The model under review builds one solid part; all positions refer to its coordinate system, in mm. Round coordinates to 2 decimals unless told otherwise and drop trailing zeros. Loops run counter-clockwise (first coordinate to the right, second up) from the corner with the lowest first, then second, coordinate; pieces in that order, holes last. Notation, with made-up numbers: (-3, 36) -> (15, 36) arc R21 cw to (15, 60) -> close; hole circle Ø6 at (-40, 34). An arc over 180 degrees is marked (long way). Use a Markdown table: item, result. Add a question column.
1) Consider section A-A on z = 0. Give the boundary of the cut face in (x, y), plus the area to 3 significant figures.
2) Insertion check: pin 1 (1.5 mm diameter, centred on x = -5, y = -2, fed in from -Z); pin 2 (2 mm diameter, centred on y = 1.5, z = 36, fed in from -X); pin 3 (2 mm diameter, centred on x = -2, z = 26.5, fed in from +Y). Each pin has a flat end and moves straight along its axis. Give the tip position at first contact, or say it passes through.
3) Wall thickness on probe 1 along X at (y, z) = (0.25, 0); probe 2 along Z at (x, y) = (0.25, 0.75); probe 3 along Z at (x, y) = (-2, -1.25): over which ranges is each line inside the solid? List them lowest first.
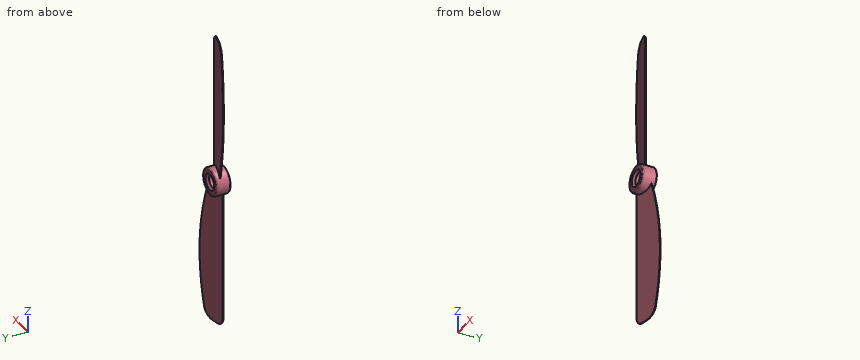
from build123d import *

# Parameters (mm, degrees)
SKETCH1_R           = 5.75
BOSS_EXTRUDE1_DEPTH = 3
BOSS_EXTRUDE2_DEPTH = 0.15
CIRPATTERN1_COUNT   = 2
SKETCH4_R           = 2.5
CUT_EXTRUDE1_DEPTH  = 7.0000001
FILLET1_R           = 0.5
CHAMFER1_SIZE       = 1


with BuildPart() as part:
    # Sketch1 → Boss-Extrude1 (new body, symmetric)
    with BuildSketch(Plane(origin=(0, 0, 0), x_dir=(1, 0, 0), z_dir=(0, 1, 0))):
        Circle(SKETCH1_R)
    extrude(amount=BOSS_EXTRUDE1_DEPTH, both=True)

    # Sketch3 → Boss-Extrude2 (add, symmetric)
    with BuildSketch(Plane(origin=(0, 0, 0), x_dir=(0.974370065, -0.224951054, 0), z_dir=(-0.224951054, -0.974370065, 0))):
        with BuildLine():
            add(Edge.make_bspline(
                [(3.543368809, 3.784271818), (1.869103712, 5.75), (-0.674853163, 5.75)],
                knots=[5.430726938, 5.430726938, 5.430726938, 6.283185307, 6.283185307, 6.283185307], degree=2, weights=[1, 0.910531227, 1]))
            Line((3.543368809, 3.784271818), (3.543368809, 60.5))
            ThreePointArc((3.543368809, 60.5), (2.664689152, 62.621320344), (0.543368809, 63.5))
            Line((0.543368809, 63.5), (-2.327174273, 63.5))
            ThreePointArc((-2.327174273, 63.5), (-5.459156928, 62.397522886), (-7.209963904, 59.576273859))
            add(Edge.make_bspline(
                [(-4.893075135, 3.784271818), (-10.655609146, 21.734523113), (-11.43974903, 40.386779673), (-7.209963904, 59.576273859)],
                knots=[0, 0, 0, 0, 0.936316624, 0.936316624, 0.936316624, 0.936316624], degree=3))
            add(Edge.make_bspline(
                [(-0.674853163, 5.75), (-3.218810038, 5.75), (-4.893075135, 3.784271818)],
                knots=[0, 0, 0, 0.852458369, 0.852458369, 0.852458369], degree=2, weights=[1, 0.910531227, 1]))
        make_face()
    boss_extrude2 = extrude(amount=BOSS_EXTRUDE2_DEPTH, both=True)

    # CirPattern1: Boss-Extrude2 ×2 about axis
    cirpattern1_axis = Axis((0, 3, 0), (0, -1, 0))
    for i in range(1, CIRPATTERN1_COUNT):
        add(boss_extrude2.rotate(cirpattern1_axis, i * 360 / CIRPATTERN1_COUNT))

    # Sketch4 → Cut-Extrude1 (cut, through all)
    with BuildSketch(Plane(origin=(0, 3, 0), x_dir=(1, 0, 0), z_dir=(0, 1, 0))):
        Circle(SKETCH4_R)
    extrude(amount=-CUT_EXTRUDE1_DEPTH, mode=Mode.SUBTRACT)

    # Fillet1
    fillet1_edges = [part.edges().sort_by_distance(p)[0] for p in [
        (-5.75, -3, 0),
        (-5.75, 3, 0),
    ]]
    fillet(fillet1_edges, radius=FILLET1_R)

    # Chamfer1
    chamfer1_edges = [part.edges().sort_by_distance(p)[0] for p in [
        (-2.5, -3, 0),
        (-2.5, 3, 0),
    ]]
    chamfer(chamfer1_edges, length=CHAMFER1_SIZE)


solid = part.part
Result set:
| question | item | result |
|---|---|---|
| 1 | outline | (-5.75, -2.5) arc R0.5 ccw to (-5.25, -3) -> (-3.5, -3) -> (-2.5, -2) -> (-2.5, 2) -> (-3.5, 3) -> (-5.25, 3) arc R0.5 ccw to (-5.75, 2.5) -> close; (2.5, -2) -> (3.5, -3) -> (5.25, -3) arc R0.5 ccw to (5.75, -2.5) -> (5.75, 2.5) arc R0.5 ccw to (5.25, 3) -> (3.5, 3) -> (2.5, 2) -> close |
| 1 | area | 36.8 mm2 |
| 2 | pin 1 | z = -3.87 |
| 2 | pin 2 | x = -9.67 |
| 2 | pin 3 | y = 0.85 |
| 3 | probe 1 | -5.75 to -2.5, 2.5 to 5.75 |
| 3 | probe 2 | -5.74 to -2.49, 2.49 to 5.74 |
| 3 | probe 3 | -5.39 to -1.5, 1.5 to 5.39 |
